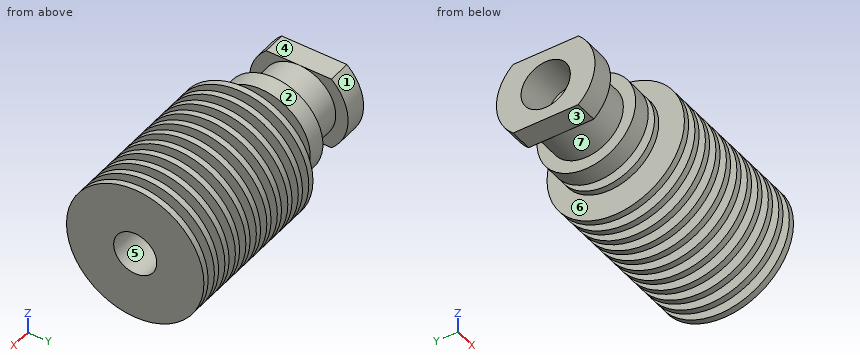
from build123d import *

# Parameters (mm, degrees)
CUT_EXTRUDE1_REACH = 44.7


with BuildPart() as part:
    # Sketch1 → Revolve1 (revolve)
    with BuildSketch(Plane.XY):
        Polygon((42.7, -3.5), (42.7, -11.15), (41.7, -11.15), (41.7, -6), (40.2, -6), (40.2, -11.15), (39.2, -11.15), (39.2, -5.868980552), (37.7, -5.868980552), (37.7, -11.15), (36.7, -11.15), (36.7, -5.737961104), (35.2, -5.737961104), (35.2, -11.15), (34.2, -11.15), (34.2, -5.606941655), (32.7, -5.606941655), (32.7, -11.15), (31.7, -11.15), (31.7, -5.475922207), (30.2, -5.475922207), (30.2, -11.15), (29.2, -11.15), (29.2, -5.344902759), (27.7, -5.344902759), (27.7, -11.15), (26.7, -11.15), (26.7, -5.213883311), (25.2, -5.213883311), (25.2, -11.15), (24.2, -11.15), (24.2, -5.082863863), (22.7, -5.082863863), (22.7, -11.15), (21.7, -11.15), (21.7, -4.951844414), (20.2, -4.951844414), (20.2, -11.15), (19.2, -11.15), (19.2, -4.820824966), (17.7, -4.820824966), (17.7, -11.15), (16.7, -11.15), (16.7, -4.689805518), (15.2, -4.689805518), (15.2, -8), (14.2, -8), (14.2, -4.689805518), (12.7, -4.689805518), (12.7, -8), (9.7, -8), (9.7, -6), (3.7, -6), (3.7, -8), (0, -8), (0, -4), (6.1, -4), (8, -2.1), (28, -2.1), (29.4, -3.5), align=None)
    revolve(axis=Axis((0, 0, 0), (1, 0, 0)))

    # Sketch2 → Cut-Extrude1 (cut, up to next)
    with BuildSketch(Plane.ZY, mode=Mode.PRIVATE) as cut_extrude1_sk1:
        with BuildLine():
            Line((6, 5.291502622), (6, -5.291502622))
            ThreePointArc((6, -5.291502622), (8, 0), (6, 5.291502622))
        make_face()
    cut_extrude1_tool1 = extrude(cut_extrude1_sk1.sketch, amount=-CUT_EXTRUDE1_REACH, mode=Mode.PRIVATE) & part.part
    add(cut_extrude1_tool1.solids().sort_by_distance((0, 0, 6.809243))[0], mode=Mode.SUBTRACT)
    # Sketch2 → Cut-Extrude1 (cut, up to next)
    with BuildSketch(Plane.ZY, mode=Mode.PRIVATE) as cut_extrude1_sk2:
        with BuildLine():
            Line((-6, 5.291502622), (-6, -5.291502622))
            ThreePointArc((-6, -5.291502622), (-8, 0), (-6, 5.291502622))
        make_face()
    cut_extrude1_tool2 = extrude(cut_extrude1_sk2.sketch, amount=-CUT_EXTRUDE1_REACH, mode=Mode.PRIVATE) & part.part
    add(cut_extrude1_tool2.solids().sort_by_distance((0, 0, -6.809243))[0], mode=Mode.SUBTRACT)


solid = part.part
Geometry: final body of the model. Coordinates: model frame, mm. Face numbers are marked on the shaded views. A direction names the side the tool comes from. Coordinates: 2 decimals unless noted, no trailing zeros. One line per item, written item: value. Start each with the question number.
1) Material intervals for L1, parallel to Y at x = 18.5, z = 0; L2, parallel to Z at x = 38.75, y = 0; L3, parallel to Y at x = 28, z = 0, sorted ascending. Write a range as from..to.
2) Draft query along Z for the marked faces 5, 6 and 7. Return one class per face: released by +Z, released by -Z, zero draft, split by the parting line, or undercut.
3) Pin query (flat end, axial travel): P1, Ø2, axis at x = 13, z = 4, coming from the -Y side; P2, Ø1.5, axis at x = 19, z = -7.5, coming from the -Y side; P3, Ø8, axis at x = 14, z = 7.5, coming from the -Y side; P4, Ø1.5, axis at x = 7, z = -8, coming from the -Y side. Return the tip coordinate at first contact, or that it passes through.
4) Reachability of the marked faces 1, 2, 3 and 4 from +Z, -Z, +X, -X, +Y, -Y: full face, straight path, thin tool, end or side. Return the list, or none.
5) Cut plane A-A (y = 9.5). Count the separate pieces of the cut face and the enclosed holes in it, then the cut area to 3 significant figures.
Evaluation:
1. L1: -4.82..-2.1, 2.1..4.82
1. L2: -5.87..-3.5, 3.5..5.87
1. L3: -5.34..-2.1, 2.1..5.34
2. face 5: undercut
2. face 6: zero draft
2. face 7: split by the parting line
3. P1: y = -7.4
3. P2: y = -8.85
3. P3: y = -10.18
3. P4: through
4. face 1: -X, +Y
4. face 2: -X
4. face 3: -Z, -X, +Y, -Y
4. face 4: +Z, -X, +Y, -Y
5. separate pieces: 11
5. enclosed holes: 0
5. area: 128 mm^2
